from build123d import *

# Parameters (mm, degrees)
SKETCH1_R     = 4.5
HEAD_DEPTH    = 1.5
SKETCH2_R     = 2.5
BODY_DEPTH    = 20
DRIVE_DEPTH   = 3
CHAMFER1_SIZE = 0.5


with BuildPart() as part:
    # Sketch1 → Head (new body)
    with BuildSketch(Plane(origin=(0, 0, 0), x_dir=(0, 0, -1), z_dir=(1, 0, 0))):
        Circle(SKETCH1_R)
    extrude(amount=HEAD_DEPTH)

    # Sketch2 → Body (add)
    with BuildSketch(Plane(origin=(1.5, 0, 0), x_dir=(0, 0, -1), z_dir=(1, 0, 0))):
        Circle(SKETCH2_R)
    extrude(amount=BODY_DEPTH)

    # Sketch3 → Drive (cut)
    with BuildSketch(Plane.ZY):
        Polygon((0, 1.732050808), (-1.5, 0.866025404), (-1.5, -0.866025404), (0, -1.732050808), (1.5, -0.866025404), (1.5, 0.866025404), align=None)
    extrude(amount=-DRIVE_DEPTH, mode=Mode.SUBTRACT)

    # Chamfer1
    chamfer1_edges = [part.edges().sort_by_distance(p)[0] for p in [
        (21.5, 0, 2.5),
    ]]
    chamfer(chamfer1_edges, length=CHAMFER1_SIZE)


solid = part.part
Geometry: final body of the model. Coordinates: model frame, mm. A direction names the side the tool comes from. Give positions to 0.01 mm unless a question says otherwise; leave off trailing zeros. Loops run counter-clockwise (first coordinate to the right, second up) from the corner with the lowest first, then second, coordinate; pieces in that order, holes last. Notation, with made-up numbers: (57, -3) - (69, -3) arc R23 cw to (69, 5) - close; hole circle Ø7 at (69, 28.25). An arc over 180 degrees is marked (long way). Answer as CSV lines item,"result". Start each with the question number.
1. Reachability of faces 5 (the face through (1, 0, 1.5)), 6 (the face through (21.5, 0, 0)), 7 (the face through (11.11, -2.44, 0.54)) from +Z, -Z, +X, -X, +Y, -Y: full face, straight path, thin tool, end or side. Return the list, or none.
2. Section D-D, the plane z = 4.25. Return loops of the section in (x, y), plus the area to 3 significant figures.
3. Draft query along Y for faces 1 (the face through (0.74, 4.46, 0.59)), 2 (the face through (1.479, -1.305, 0.74)), 3 (the face through (1.5, -2, -2)), 4 (the face through (1, 0, -1.5)). Return one class per face: released by +Y, released by -Y, zero draft, split by the parting line, or undercut.
4. Pin query (flat end, axial travel): P1, Ø4, axis at x = 5.5, y = -3, coming from the +Z side; P2, Ø4, axis at x = 15.5, z = 3.5, coming from the +Y side; P3, Ø0.9, axis at y = 0, z = 0.5, coming from the -X side. Return the tip coordinate at first contact, or that it passes through.
5. Section C-C, the plane z = -3.25. Return loops of the section in (x, y).
6. Section B-B, the plane x = 12. Return loops of the section in (y, z), plus the area to 3 significant figures.
7. Section A-A, the plane y = 0. Return loops of the section in (x, z).
8. Ray query, L1, parallel to Y at x = 5.75, z = -2; L2, parallel to X at y = 1, z = -2.75; L3, parallel to X at y = 0.5, z = -0.75. Return the intervals inside material, ascending.
Answers:
1,face 5,"-X"
1,face 6,"+Z, -Z, +X, +Y, -Y"
1,face 7,"+X"
2,outline,"(0, -1.48) - (1.5, -1.48) - (1.5, 1.48) - (0, 1.48) - close"
2,area,"4.44 mm2"
3,face 1,"split by the parting line"
3,face 2,"undercut"
3,face 3,"zero draft"
3,face 4,"undercut"
4,P1,"stops at z = 2.29"
4,P2,"stops at y = 2"
4,P3,"stops at x = 3"
5,outline,"(0, -3.11) - (1.5, -3.11) - (1.5, 3.11) - (0, 3.11) - close"
6,outline,"circle Ø5 at (0, 0)"
6,area,"19.6 mm2"
7,outline,"(0, -4.5) - (1.5, -4.5) - (1.5, -2.5) - (21, -2.5) - (21.5, -2) - (21.5, 2) - (21, 2.5) - (1.5, 2.5) - (1.5, 4.5) - (0, 4.5) - (0, 1.5) - (3, 1.5) - (3, -1.5) - (0, -1.5) - close"
8,L1,"y = -1.5 to 1.5"
8,L2,"x = 0 to 1.5"
8,L3,"x = 3 to 21.5"
